The model under review builds one solid part; all positions refer to its coordinate system, in mm. Give positions to 0.01 mm unless a question says otherwise; leave off trailing zeros. Loops run counter-clockwise (first coordinate to the right, second up) from the corner with the lowest first, then second, coordinate; pieces in that order, holes last. Notation, with made-up numbers: (78.5, 87) - (128.5, 87) arc R26 ccw to (128.5, 118) - close; hole circle Ø6 at (3.5, 26.25). An arc over 180 degrees is marked (long way). Answer as a JSON object with one key per item and string values.
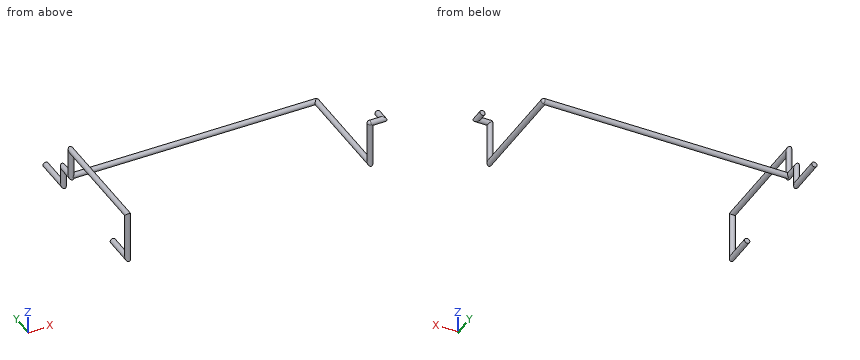
from build123d import *

# Parameters (mm, degrees)
F0_R  = 7.5
F3_R  = 7.5
F7_R  = 7.5
F11_R = 7.5


with BuildPart() as f2:
    # F2: sweep along a path in F1
    with BuildLine(Plane.YZ) as f2_path:
        Line((0, 0), (-80.781, 0))
        Line((-80.781, 0), (-80.781, 134.381))
        Line((-80.781, 134.381), (228, 134.381))
        Line((228, 134.381), (228, 54.381))
        Line((228, 54.381), (270.740032196, 54.381))
        Line((270.740032196, 54.381), (270.740032196, 0))
        Line((270.740032196, 0), (367.740032196, 0))
    # F0 (on Front) → F2 (sweep)
    with BuildSketch(Plane.XZ):
        Circle(F0_R)
    sweep(path=f2_path.line, transition=Transition.RIGHT)

    # F5: sweep along a path in F4
    with BuildLine(Plane.XZ) as f5_path:
        Line((0, 0), (695, 0))
    # F3 (on Right) → F5 (sweep)
    with BuildSketch(Plane.YZ):
        with Locations((228, 54.381)):
            Circle(F3_R)
    sweep(path=f5_path.line)

    # F9: sweep along a path in F8
    with BuildLine(Plane.YZ) as f9_path:
        Line((228, 54.381), (-65.727, 54.381))
        Line((-65.727, 54.381), (-65.727, 176.355))
    # F7 (on offset) → F9 (sweep)
    with BuildSketch(Plane.XZ.offset(-228)):
        with Locations((695, 54.381)):
            Circle(F7_R)
    sweep(path=f9_path.line, transition=Transition.RIGHT)

    # F13: sweep along a path in F12
    with BuildLine(Plane.XY) as f13_path:
        Line((695, -65.727), (732, -65.727))
        Line((732, -65.727), (732, -35.727))
    # F11 (on offset) → F13 (sweep)
    with BuildSketch(Plane.YZ.offset(695)):
        with Locations((-65.727, 176.355)):
            Circle(F11_R)
    sweep(path=f13_path.line, transition=Transition.RIGHT)

    # F9_face (on face) → F14 (revolve)
    with BuildSketch(Plane(origin=(691.8169011382, -65.727, 176.355), x_dir=(1, 0, 0), z_dir=(0, 0, 1))):
        with BuildLine():
            Line((3.1830988618, -7.5), (3.1830988618, 7.5))
            ThreePointArc((3.1830988618, 7.5), (-4.3169011382, 0), (3.1830988618, -7.5))
        make_face()
    revolve(axis=Axis((695, -65.727, 176.355), (0, -1, 0)))

    # F9_face1 (on face) → F15 (revolve)
    with BuildSketch(Plane(origin=(698.1830988618, 228, 54.381), x_dir=(-1, 0, 0), z_dir=(0, 1, 0))):
        with BuildLine():
            ThreePointArc((-4.3169011382, 0), (-2.1202019971, -5.3033008589), (3.1830988618, -7.5))
            Line((3.1830988618, -7.5), (3.1830988618, 7.5))
            ThreePointArc((3.1830988618, 7.5), (-2.1202019971, 5.3033008589), (-4.3169011382, 0))
        make_face()
    revolve(axis=Axis((695, 228, 54.381), (0, 0, 1)))


solid = f2.part
Q1. Consider section B-B, the plane y = 11.5. State the section outline as (x, z) points.
Results:
{"outline": "circle Ø15 at (0, 134.38); circle Ø15 at (695, 54.38)"}
Q2. To check wall thickness, follow probe 1 along X at (y, z) = (8, 48.5); probe 2 along Z at (x, y) = (701, 99); probe 3 along X at (y, z) = (144, 132). State the ranges of each line that lie inside material, in increasing order. Write a range as [from, to].
Results:
{"probe 1": "x = [690.35, 699.65]", "probe 2": "z = [49.88, 58.88]", "probe 3": "x = [-7.11, 7.11]"}
Q3. Clearance check with flat-ended pins moving along their axes: pin 1 Ø1 at (y, z) = (-33, 125.5) entering from -X; pin 2 Ø5 at (x, z) = (157.5, 48.5) entering from +Y; pin 3 Ø4.5 at (x, z) = (730.5, 176) entering from +Y. State where each tip first meets the part, or that it passes through.
Results:
{"pin 1": "passes through", "pin 2": "stops at y = 234.69", "pin 3": "stops at y = -35.73"}
Q4. Consider section A-A, the plane z = 0. State the section outline as (x, y) points.
Results:
{"outline": "(-7.5, -80.78) arc R7.5 ccw to (7.5, -80.78) - (7.5, 0) - (-7.5, 0) - close; (-7.5, 270.74) arc R7.5 ccw to (7.5, 270.74) - (7.5, 367.74) - (-7.5, 367.74) - close"}
Q5. Consider section D-D, the plane x = 162.5. State the section outline as (y, z) points.
Results:
{"outline": "circle Ø15 at (228, 54.38)"}
Q6. Consider section C-C, the plane z = 92.5. State the section outline as (x, y) points.
Results:
{"outline": "circle Ø15 at (0, -80.78); circle Ø15 at (0, 228); circle Ø15 at (695, -65.73)"}
